from build123d import *

# Parameters (mm, degrees)
BOSS_EXTRUDE1_DEPTH      = 30
BOSS_EXTRUDE1_DEPTH_BACK = 10
SKETCH1_W                = 150
SKETCH1_H                = 95
SKETCH1_R                = 7


with BuildPart() as part:
    # Sketch1 → Boss-Extrude1 (new, two sides: drawn at the far end of the back side and taken through both)
    with BuildSketch(Plane(origin=(0, 0, 0), x_dir=(1, 0, 0), z_dir=(0, 1, 0)).offset(-BOSS_EXTRUDE1_DEPTH_BACK)):
        Rectangle(SKETCH1_W, SKETCH1_H)
        with Locations(Location((-50, 31.666666667, 0), (0, 0, 270))):
            Circle(SKETCH1_R, mode=Mode.SUBTRACT)
        with Locations(Location((50, 31.666666667, 0), (0, 0, 270))):
            Circle(SKETCH1_R, mode=Mode.SUBTRACT)
        with Locations(Location((-58.389104437, -36.979766144, 0), (0, 0, 270))):
            Circle(SKETCH1_R, mode=Mode.SUBTRACT)
        with Locations(Location((58.389104437, -36.979766144, 0), (0, 0, 270))):
            Circle(SKETCH1_R, mode=Mode.SUBTRACT)
        with BuildLine():
            Line((-50, 10), (50, 10))
            ThreePointArc((50, 10), (60, 0), (50, -10))
            Line((50, -10), (-50, -10))
            ThreePointArc((-50, -10), (-60, 0), (-50, 10))
        make_face(mode=Mode.SUBTRACT)
    extrude(amount=BOSS_EXTRUDE1_DEPTH + BOSS_EXTRUDE1_DEPTH_BACK)


solid = part.part
Verification items for the finished model (mm, model axes). A direction names the side the tool comes from. Round coordinates to 2 decimals unless told otherwise and drop trailing zeros. Write each loop counter-clockwise with the first axis right and the second up, starting at its lowest first coordinate (ties: lowest second). Pieces come first, ordered by that corner, then holes.
(1) Section check D-D (y = 25). Enter the section's corners in (x, z), plus the area to 3 significant figures.
Returned:
outline: (-75, -47.5) - (75, -47.5) - (75, 47.5) - (-75, 47.5) - close; hole circle Ø14 at (-58.39, 36.98); hole circle Ø14 at (-50, -31.67); hole (-50, -10) - (50, -10) arc R10 ccw to (50, 10) - (-50, 10) arc R10 ccw to start; hole circle Ø14 at (50, -31.67); hole circle Ø14 at (58.39, 36.98)
area: 11,300 mm2
(2) Material ranges on line 1 (Z direction, x = 33.5, y = 15); line 2 (X direction, y = 4, z = 37.5); line 3 (Z direction, x = 54, y = 1), recorded low to high.
Returned:
line 1: z = -47.5 to -10, 10 to 47.5
line 2: x = -75 to -65.37, -51.41 to 51.41, 65.37 to 75
line 3: z = -47.5 to -37.41, -25.92 to -9.17, 9.17 to 31.53, 42.43 to 47.5
(3) Access from +Z, -Z, +X, -X, +Y, -Y to the whole of each face (thin tool, end or side, straight path). Record for faces 5 (the flat face through (-1, 10, 47.5)), 6 (the flat face through (-1, 10, -10)).
Returned:
face 5: +Z, +X, -X, +Y, -Y
face 6: +Y, -Y
(4) Mould release check, pull along X, two halves, no side actions. Record for faces 1 (the cylindrical face through (-64.6, 9.72, 40.21)), 2 (the cylindrical face through (56.94, 9.72, -32.58)), 3 (the flat face through (75, 10, 1)), 4 (the flat face through (-1, 30, -11)): pulls with the +X half, pulls with the -X half, needs draft (parallel to the pull), parting line crosses it, or undercut.
Returned:
face 1: undercut
face 2: undercut
face 3: pulls with the +X half
face 4: needs draft
(5) Section check C-C (z = -36). Enter the section's corners in (x, y), plus the area to 3 significant figures.
Returned:
outline: (-75, -10) - (-55.5, -10) - (-55.5, 30) - (-75, 30) - close; (-44.5, -10) - (44.5, -10) - (44.5, 30) - (-44.5, 30) - close; (55.5, -10) - (75, -10) - (75, 30) - (55.5, 30) - close
area: 5,120 mm2
(6) Section check A-A (z = 0). Enter the section's corners in (x, y), plus the area to 3 significant figures.
Returned:
outline: (-75, -10) - (-60, -10) - (-60, 30) - (-75, 30) - close; (60, -10) - (75, -10) - (75, 30) - (60, 30) - close
area: 1,200 mm2
(7) Section check B-B (x = -36). Enter the section's corners in (y, z).
Returned:
outline: (-10, -47.5) - (30, -47.5) - (30, -10) - (-10, -10) - close; (-10, 10) - (30, 10) - (30, 47.5) - (-10, 47.5) - close
(8) Depth check by flat-ended pin: pin 1 Ø8.5 at (x, z) = (58.39, 36.98) entering from -Y. Enter the tip coordinate at first touch or a pass-through.
Returned:
pin 1: passes through
